```python
from build123d import *

# Parameters (mm, degrees)
F0_R     = 31.75
F1_DEPTH = 25.4
F3_SIZE  = 5.08
F4_R     = 26.67
F5_DEPTH = 25.4
F6_R     = 5.19146
F6_R_2   = 7.272236
F6_R_3   = 6.757556
F6_R_4   = 4.56385
F7_DEPTH = 17.78


with BuildPart() as f1:
    # F0 (on Front) → F1 (new body)
    with BuildSketch(Plane.XZ):
        Circle(F0_R)
    extrude(amount=F1_DEPTH)

    # F3
    f3_edges = [f1.edges().sort_by_distance(p)[0] for p in [
        (-31.75, 0, 0),
    ]]
    chamfer(f3_edges, length=F3_SIZE)

    # F4 (on face) → F5 (join)
    with BuildSketch(Plane(origin=(0, 0, 0), x_dir=(-1, 0, 0), z_dir=(0, 1, 0))):
        Circle(F4_R)
    extrude(amount=F5_DEPTH)

    # F6 (on face) → F7 (join)
    with BuildSketch(Plane(origin=(0, 25.4, 0), x_dir=(-1, 0, 0), z_dir=(0, 1, 0))):
        with Locations((0, 17.68492)):
            Circle(F6_R)
        with Locations((-17.257057, 0)):
            Circle(F6_R_2)
        with Locations((0, -18.255401)):
            Circle(F6_R_3)
        with Locations((16.971817, 0)):
            Circle(F6_R_4)
    extrude(amount=F7_DEPTH)


solid = f1.part
```
Part model, mm, in its own coordinate system. A direction names the side the tool comes from. Round coordinates to 2 decimals unless told otherwise and drop trailing zeros. Write each loop counter-clockwise with the first axis right and the second up, starting at its lowest first coordinate (ties: lowest second). Pieces come first, ordered by that corner, then holes. Notation, with made-up numbers: M 71,24 L 82,24 A28 cw 82,46 Z; hole C -34.5,49.5 d6. An arc over 180 degrees is marked long. Answer as CSV lines item,"result". Start each with the question number.
1) Mould opens along Z. For faces 3 (the face through (0, 43.18, -18)), 4 (the face through (24.522, 34.166, 0.32)), 5 (the face through (1.465, 34.166, -24.852)) say: +Z half, -Z half, draft (parallel to the pull), parting line (faces both ways), or undercut.
2) Band-saw the part on D-D (y = -16). List the corners of the cut face in (x, z), then the cut area to 3 significant figures.
3) Drill centre lines: L1, parallel to Y at x = -8, z = 22; L2, parallel to Z at x = 0.5, y = 28.5; L3, parallel to Z at x = 0, y = 23.5. Where is each one in solid material? Low to high.
4) Drop flat-ended pins along their axis: pin 1 (5 mm diameter, centred on y = -9.5, z = -8, fed in from -X); pin 2 (4 mm diameter, centred on x = -12.5, y = 3, fed in from +Z); pin 3 (5 mm diameter, centred on y = -5, z = 22.5, fed in from +X). Give the stop position or say it passes through.
5) Band-saw the part on B-B (x = 0). List the corners of the cut face in (y, z).
6) Which spindle directions (+Z, -Z, +X, -X, +Y, -Y) get a long thin tool onto all of the face, cutting with end or side? Do faces 1 (the face through (-12.412, 34.166, 0.201)), 2 (the face through (-6.883, -15.098, -30.995)). Say none if no direction does.
7) Band-saw the part on A-A (z = 0). List the corners of the cut face in (x, y), then the cut area to 3 significant figures.
8) Band-saw the part on C-C (y = 13). List the corners of the cut face in (x, z).
Worked out:
1,face 3,"draft"
1,face 4,"parting line"
1,face 5,"undercut"
2,outline,"C 0,0 d63.5"
2,area,"3,170 mm²"
3,L1,"-25.4 to 25.4"
3,L2,"-24.99 to -11.52, 12.52 to 22.85"
3,L3,"-26.67 to 26.67"
4,pin 1,"x = -31.27"
4,pin 2,"z = 24.52"
4,pin 3,"x = 24.66"
5,outline,"M -25.4,-31.75 L -5.08,-31.75 L 0,-26.67 L 25.4,-26.67 L 25.4,-25.01 L 43.18,-25.01 L 43.18,-11.5 L 25.4,-11.5 L 25.4,12.49 L 43.18,12.49 L 43.18,22.88 L 25.4,22.88 L 25.4,26.67 L 0,26.67 L -5.08,31.75 L -25.4,31.75 Z"
6,face 1,"+Y"
6,face 2,"+Y, -Y"
7,outline,"M -31.75,-25.4 L 31.75,-25.4 L 31.75,-5.08 L 26.67,0 L 26.67,25.4 L 24.53,25.4 L 24.53,43.18 L 9.98,43.18 L 9.98,25.4 L -12.41,25.4 L -12.41,43.18 L -21.54,43.18 L -21.54,25.4 L -26.67,25.4 L -26.67,0 L -31.75,-5.08 Z"
7,area,"3,360 mm²"
8,outline,"C 0,0 d53.34"
